Can you work these out from the model? Positions are in its coordinate system, mm. A direction names the side the tool comes from. Give positions to 0.01 mm unless a question says otherwise; leave off trailing zeros. Loops run counter-clockwise (first coordinate to the right, second up) from the corner with the lowest first, then second, coordinate; pieces in that order, holes last. Notation, with made-up numbers: (47, -5.75) -> (59, -5.75) arc R22 ccw to (59, 1.25) -> close; hole circle Ø4 at (9, 1). An arc over 180 degrees is marked (long way). Use CSV: the item, a comma, the result in double quotes.
Autodesk Inventor part; units mm, degrees
ref_plane "YZ Plane" through (0, 0, 0) normal (1, 0, 0) x (0, 1, 0)
ref_plane "XZ Plane" through (0, 0, 0) normal (0, 1, 0) x (-1, 0, 0)
ref_plane "XY Plane" through (0, 0, 0) normal (0, 0, 1) x (1, 0, 0)
sketch "Sketch1" plane through (0, 0, 0) normal (0, 0, 1) x (1, 0, 0)
  line L0 (-15.875, -31.75) -> (15.875, -31.75)
  line L1 (15.875, -31.75) -> (15.875, 31.75)
  line L2 (15.875, 31.75) -> (-15.875, 31.75)
  line L3 (-15.875, 31.75) -> (-15.875, -31.75)
  line L4 (-15.875, -31.75) -> (15.875, 31.75) construction
  line L5 (15.875, -31.75) -> (-15.875, 31.75) construction
  point P0 (0, 0)
  dimension "height" = 63.5
  dimension "width" = 31.75
extrude "Extrusion1" add sketch "Sketch1" against normal blind 12.7
sketch "Sketch3" plane through (0, 0, 0) normal (0, 0, 1) x (1, 0, 0)
  line L0 (-15.875, -9.525) -> (15.875, -9.525)
  line L1 (15.875, -9.525) -> (15.875, 9.525)
  line L2 (15.875, 9.525) -> (-15.875, 9.525)
  line L3 (-15.875, 9.525) -> (-15.875, -9.525)
  line L4 (-15.875, -9.525) -> (15.875, 9.525) construction
  line L5 (15.875, -9.525) -> (-15.875, 9.525) construction
  line L6 (15.875, 31.75) -> (-15.875, 31.75)
  point P0 (0, 0)
  dimension "Channel_Width" = 19.05
  dimension "d52" = 31.75
extrude "Extrusion3" add sketch "Sketch3" along normal blind 50.8
sketch "Sketch6" plane through (15.875, -31.75, -12.7) normal (1, 0, 0) x (0, 0, -1)
  line L0 (-12.7, 31.75) -> (-63.5, 31.75) construction
  line L1 (-63.5, 22.225) -> (-63.5, 41.275) construction
  line L2 (-12.7, 41.275) -> (-12.7, 63.5) construction
  point P0 (-50.8, 31.75)
  dimension "d53" = 38.1
hole "Hole5" at (15.875, 0, 38.1) direction (-1, 0, 0) diameter 9.7282 end through all
sketch "Sketch13" plane through (15.875, -31.75, -12.7) normal (1, 0, 0) x (0, 0, -1)
  line L0 (-12.7, 63.5) -> (0, 63.5)
  line L1 (0, 0) -> (-6.35, 0)
  line L2 (-6.35, 0) -> (-6.35, 63.5)
  line L3 (-6.35, 63.5) -> (0, 63.5)
  line L4 (0, 63.5) -> (0, 0)
  point P0 (-12.7, 31.75)
  dimension "d98" = 6.35
extrude "Extrusion5" cut sketch "Sketch13" against normal through all
sketch "Sketch14" plane through (-15.875, -31.75, 0) normal (-1, 0, 0) x (0, 0, 1)
  line L0 (0, 0) -> (-6.35, 0)
  line L1 (0, 0) -> (0, 22.225)
  line L2 (-6.35, 0) -> (0, 0)
  line L3 (0, 0) -> (0, 6.604)
  line L4 (0, 6.604) -> (-6.35, 6.604)
  line L5 (-6.35, 6.604) -> (-6.35, 0)
  point P0 (0, 31.75)
  dimension "d101" = 6.604
extrude "Extrusion6" cut sketch "Sketch14" against normal through all
sketch "Sketch15" plane through (-15.875, 9.525, 0) normal (0, 1, 0) x (1, 0, 0)
  line L0 (31.75, -50.8) -> (0, -50.8)
  point P0 (15.875, 0)
  point P1 (15.875, -25.4)
  dimension "d104" = 25.4
hole "Hole11" at (0, 9.525, 25.4) direction (0, -1, 0) diameter 4.9784 end through all
sketch "Sketch11" plane through (0, 0, 50.8) normal (0, 0, 1) x (1, 0, 0)
  point P0 (0, 0)
hole "Hole12" at (0, 0, 50.8) direction (0, 0, -1) diameter 4.9784 depth 12.7 tip angle 118
sketch "Sketch10" plane through (0, 0, 50.8) normal (0, 0, 1) x (1, 0, 0)
  point P0 (0, 0)
sketch "Sketch12" plane through (-15.875, -9.525, 0) normal (0, -1, 0) x (1, 0, 0)
  point P0 (15.875, 15.875)
equation "\"d52\" = width"
properties part number "Support For Arms" material "Aluminum 6061"
(1) If I drill on L1, parallel to Y at x = -2.5, z = 38.1 (3 decimals); L2, parallel to X at y = 4.75, z = 25.4 (3 decimals); L3, parallel to Z at x = 0, y = 4.5, over which ranges is the centre line in solid material (lowest first)? Write a range as from..to.
Answer sheet:
L1,"y = -9.525..-4.864, 4.864..9.525"
L2,"x = -15.875..-2.489, 2.489..15.875"
L3,"z = -6.35..22.91, 27.89..36.25, 39.95..50.8"
(2) We'd pull the mould along Y, two halves only. Please class faces 3 (the face through (-3, 9.525, 25)), 4 (the face through (-0.109, 2.487, 46.48)), 5 (the face through (0, -17, 0)), 6 (the face through (3, -9.525, 25)): released by +Y, released by -Y, zero draft, split by the parting line, or undercut.
Answer sheet:
face 3,"released by +Y"
face 4,"undercut"
face 5,"zero draft"
face 6,"released by -Y"
(3) If we section it at C-C, the plane x = 0: Write out the boundary of the cut face in (y, z) (3 decimals), then the cut area to 3 significant figures.
Answer sheet:
outline,"(-25.146, -6.35) -> (31.75, -6.35) -> (31.75, 0) -> (9.525, 0) -> (9.525, 22.911) -> (-9.525, 22.911) -> (-9.525, 0) -> (-25.146, 0) -> close; (-9.525, 27.889) -> (9.525, 27.889) -> (9.525, 50.8) -> (2.489, 50.8) -> (2.489, 42.279) arc R4.864 cw (long way) to (-2.489, 42.279) -> (-2.489, 50.8) -> (-9.525, 50.8) -> close"
area,"1,120 mm2"
(4) If we section it at D-D, the plane x = 8: Write out the boundary of the cut face in (y, z) (3 decimals), then the cut area to 3 significant figures.
Answer sheet:
outline,"(-25.146, -6.35) -> (31.75, -6.35) -> (31.75, 0) -> (9.525, 0) -> (9.525, 50.8) -> (-9.525, 50.8) -> (-9.525, 0) -> (-25.146, 0) -> close; hole circle Ø9.728 at (0, 38.1)"
area,"1,250 mm2"
(5) Which directions (+Z, -Z, +X, -X, +Y, -Y) give clear straight access to the entire face, cutting with the end or side of a thin tool? Please do faces 1 (the face through (0, 21, 0)), 2 (the face through (0, -25.146, -3)).
Answer sheet:
face 1,"+Z, +X, -X, +Y"
face 2,"+Z, -Z, +X, -X, -Y"
(6) If we section it at A-A, the plane y = 0: Write out the boundary of the cut face in (x, z) (3 decimals), then the cut area to 3 significant figures.
Answer sheet:
outline,"(-15.875, -6.35) -> (15.875, -6.35) -> (15.875, 33.236) -> (-15.875, 33.236) -> close; (-15.875, 42.964) -> (-2.489, 42.964) -> (-2.489, 50.8) -> (-15.875, 50.8) -> close; (2.489, 42.964) -> (15.875, 42.964) -> (15.875, 50.8) -> (2.489, 50.8) -> close; hole circle Ø4.978 at (0, 25.4)"
area,"1,450 mm2"
(7) Will these pins go through, and if not, where does the flat tip stop? pin 1 Ø6.5 at (x, y) = (-1, 22) entering from +Z; pin 2 Ø9.5 at (x, z) = (4, 27.5) entering from +Y (3 decimals); pin 3 Ø3 at (x, y) = (0, 0) entering from +Z.
Answer sheet:
pin 1,"stops at z = 0"
pin 2,"stops at y = 9.525"
pin 3,"stops at z = 33.47"
(8) If we section it at B-B, the plane z = 25.4: Write out the boundary of the cut face in (x, y) (3 decimals), then the cut area to 3 significant figures.
Answer sheet:
outline,"(-15.875, -9.525) -> (-2.489, -9.525) -> (-2.489, 9.525) -> (-15.875, 9.525) -> close; (2.489, -9.525) -> (15.875, -9.525) -> (15.875, 9.525) -> (2.489, 9.525) -> close"
area,"510 mm2"
